```python
from build123d import *

# Parameters (mm, degrees)
SKETCH_2_R          = 5
EXTRUDE_1_DEPTH     = 20
SKETCH_3_R          = 8
EXTRUDE_2_DEPTH     = 7
SKETCH_4_R          = 4
EXTRUDE_3_DEPTH     = 13.25
CUT_EXTRUDE_1_DEPTH = 3
CHAMFER_1_SIZE      = 0.5
SKETCH_6_R          = 4
SKETCH_6_R_2        = 3.5
CUT_EXTRUDE_2_DEPTH = 1


with BuildPart() as part:
    # 草图2 → 凸台-拉伸1 (new body)
    with BuildSketch(Plane(origin=(0, 0, 0), x_dir=(1, 0, 0), z_dir=(0, 1, 0))):
        with Locations(Location((0, 0, 0), (0, 0, 270))):
            Circle(SKETCH_2_R)
    extrude(amount=EXTRUDE_1_DEPTH)

    # 草图3 → 凸台-拉伸2 (add)
    with BuildSketch(Plane.XZ):
        with Locations(Location((0, 0, 0), (0, 0, 270))):
            Circle(SKETCH_3_R)
    extrude(amount=EXTRUDE_2_DEPTH)

    # 草图4 → 凸台-拉伸3 (add)
    with BuildSketch(Plane(origin=(0, 20, 0), x_dir=(1, 0, 0), z_dir=(0, 1, 0))):
        with Locations(Location((0, 0, 0), (0, 0, 270))):
            Circle(SKETCH_4_R)
    extrude(amount=EXTRUDE_3_DEPTH)

    # 草图5 → 切除-拉伸1 (cut)
    with BuildSketch(Plane.XZ.offset(7)):
        Polygon((0.295951976, 5.999509568), (-5.047751708, 3.256056713), (-5.343703684, -2.743452854), (-0.295951976, -5.999509568), (5.047751708, -3.256056713), (5.343703684, 2.743452854), align=None)
    extrude(amount=-CUT_EXTRUDE_1_DEPTH, mode=Mode.SUBTRACT)

    # 倒角1
    chamfer_1_edges = [part.edges().sort_by_distance(p)[0] for p in [
        (0, 33.25, -4),
    ]]
    chamfer(chamfer_1_edges, length=CHAMFER_1_SIZE)

    # 草图6 → 切除-拉伸2 (cut)
    with BuildSketch(Plane(origin=(0, 20, 0), x_dir=(1, 0, 0), z_dir=(0, 1, 0))):
        with Locations(Location((0, 0, 0), (0, 0, 270))):
            Circle(SKETCH_6_R)
        with Locations(Location((0, 0, 0), (0, 0, 270))):
            Circle(SKETCH_6_R_2, mode=Mode.SUBTRACT)
    extrude(amount=CUT_EXTRUDE_2_DEPTH, mode=Mode.SUBTRACT)


solid = part.part
```
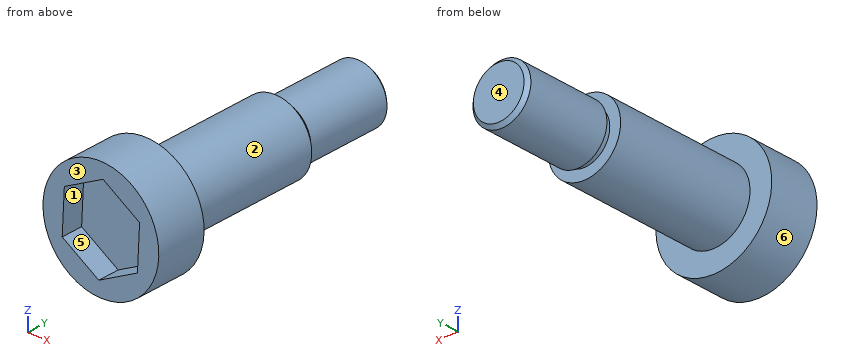
For this review, take the finished solid that the model builds, in its own axes (mm). Face numbers are marked on the shaded views. A direction names the side the tool comes from. Round coordinates to 2 decimals unless told otherwise and drop trailing zeros. Loops run counter-clockwise (first coordinate to the right, second up) from the corner with the lowest first, then second, coordinate; pieces in that order, holes last.
Q1. To check wall thickness, follow line 1 along Y through (x, z) = (4.5, -4.75); line 2 along Y through (x, z) = (1.5, -4.5); line 3 along Y through (x, z) = (3.25, -2). State the ranges of each line that lie inside material, in increasing order.
Result sheet:
line 1: y = -7 to 0
line 2: y = -4 to 20
line 3: y = -4 to 20, 21 to 32.93
Q2. Add section C-C on x = 4.5. Write out the cut boundary in (y, z), plus the area to 3 significant figures.
Result sheet:
outline: (-7, -6.61) - (0, -6.61) - (0, -2.18) - (20, -2.18) - (20, 2.18) - (0, 2.18) - (0, 6.61) - (-7, 6.61) - (-7, 3.29) - (-4, 3.29) - (-4, -3.54) - (-7, -3.54) - close
area: 159 mm2
Q3. Add section A-A on z = 0. Write out the cut boundary in (x, y).
Result sheet:
outline: (-8, -7) - (-5.21, -7) - (-5.21, -4) - (5.21, -4) - (5.21, -7) - (8, -7) - (8, 0) - (5, 0) - (5, 20) - (3.5, 20) - (3.5, 21) - (4, 21) - (4, 32.75) - (3.5, 33.25) - (-3.5, 33.25) - (-4, 32.75) - (-4, 21) - (-3.5, 21) - (-3.5, 20) - (-5, 20) - (-5, 0) - (-8, 0) - close
Q4. Insertion check: pin 1 Ø3 at (x, z) = (0.5, -0.5) entering from -Y; pin 2 Ø6 at (x, y) = (3, 14.5) entering from +Z; pin 3 Ø1 at (x, y) = (2.5, 14) entering from -Z. Each pin has a flat end and moves straight along its axis. Give the tip position at first contact, or say it passes through.
Result sheet:
pin 1: stops at y = -4
pin 2: stops at z = 5
pin 3: stops at z = -4.58
Q5. Add section B-B on y = -0.5. Write out the cut boundary in (x, z), plus the area to 3 significant figures.
Result sheet:
outline: circle Ø16 at (0, 0)
area: 201 mm2
Q6. Add section D-D on z = 4.5. Write out the cut boundary in (x, y), plus the area to 3 significant figures.
Result sheet:
outline: (-6.61, -7) - (-2.62, -7) - (-2.62, -4) - (2.62, -4) - (2.62, -7) - (6.61, -7) - (6.61, 0) - (2.18, 0) - (2.18, 20) - (-2.18, 20) - (-2.18, 0) - (-6.61, 0) - close
area: 164 mm2
Q7. Machinability: for the marked faces 1, 2 and 3, which of the approach directions +Z, -Z, +X, -X, +Y, -Y give a long, thin tool a straight path to every point of the face, cutting with its end or side? Answer none if there is none.
Result sheet:
face 1: -Y
face 2: +Y
face 3: +Z, -Z, +X, -X, -Y
Q8. Mouldability with a two-part tool opening along X and no side actions: class the marked faces 4, 5 and 6 as +X half, -X half, draft (parallel to the pull), parting line (faces both ways), or undercut.
Result sheet:
face 4: draft
face 5: undercut
face 6: parting line
